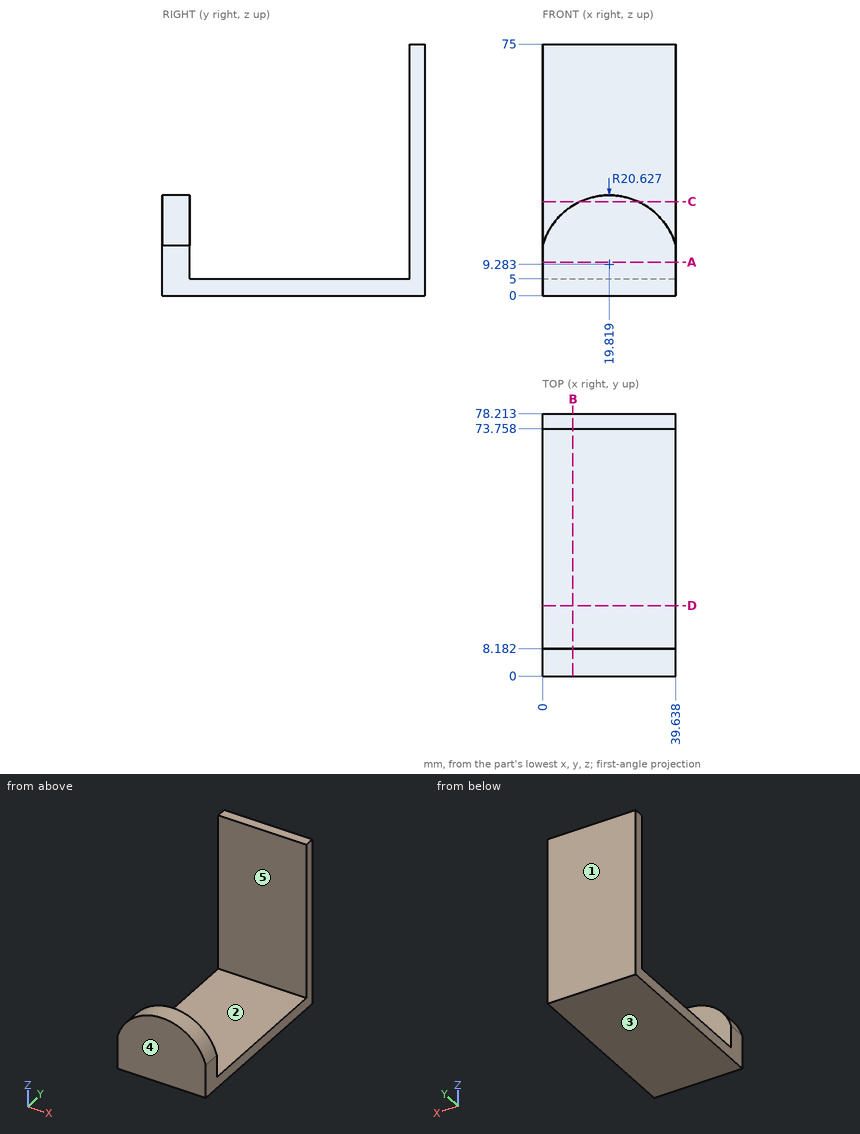
Geometry check sheet. Reference: drawing and pictorial views, mm from the part's lowest x, y, z. A direction names the side the tool comes from. Coordinates: 2 decimals unless noted, no trailing zeros. Order: outer loops, then holes, each group sorted by start corner. A loop starts at its lowest first (then second) coordinate and runs counter-clockwise, first axis right, second up. Notation, with made-up numbers: M -4.75,26.25 L 2.25,26.25 A28 ccw 2.25,63.25 Z; hole C -6,3 d9. An arc over 180 degrees is marked long. Return JSON: item names as keys, results as strings.
1) Cross-section at B-B, the plane x = 9. Record the boundary of the cut face in (y, z) (1 decimal).
Answer list:
{"outline": "M 0,0 L 78.2,0 L 78.2,75 L 73.8,75 L 73.8,5 L 8.2,5 L 8.2,26.8 L 0,26.8 Z"}
2) Cross-section at D-D, the plane y = 21. Record the boundary of the cut face in (x, z), and give its area (3 significant figures).
Answer list:
{"outline": "M 0,0 L 39.64,0 L 39.64,5 L 0,5 Z", "area": "198 mm2"}
3) Access from +Z, -Z, +X, -X, +Y, -Y to the whole of each face (thin tool, end or side, straight path). Record for the marked faces 1 and 2.
Answer list:
{"face 1": "+Z, -Z, +X, -X, +Y", "face 2": "+Z, +X, -X"}
4) Thickness scan on L1, parallel to Y at x = 19.5, z = 26.5; L2, parallel to Z at x = 21, y = 12; L3, parallel to Y at x = 26.5, z = 47.5. Record the ranges inside material, lowest first. Write a range as [from, to].
Answer list:
{"L1": "[0, 8.18], [73.76, 78.21]", "L2": "[0, 5]", "L3": "[73.76, 78.21]"}
5) Release check for a two-part mould opening along Y. For the marked faces 3, 4 and 5 record: +Y half, -Y half, draft (parallel to the pull), parting line (faces both ways), or undercut.
Answer list:
{"face 3": "draft", "face 4": "-Y half", "face 5": "undercut"}
6) Gauge pin test, flat end, axial feed: pin 1 (3 mm diameter, centred on x = 32.5, y = 26, fed in from +Z). Record the tip position at first contact, or that the pin passes through.
Answer list:
{"pin 1": "z = 5"}
7) Cross-section at C-C, the plane z = 28. Record the boundary of the cut face in (x, y).
Answer list:
{"outline": "M 0,73.76 L 39.64,73.76 L 39.64,78.21 L 0,78.21 Z; M 11.15,0 L 28.49,0 L 28.49,8.18 L 11.15,8.18 Z"}
8) Cross-section at A-A, the plane z = 10. Record the boundary of the cut face in (x, y), and give its area (3 significant figures).
Answer list:
{"outline": "M 0,0 L 39.64,0 L 39.64,8.18 L 0,8.18 Z; M 0,73.76 L 39.64,73.76 L 39.64,78.21 L 0,78.21 Z", "area": "501 mm2"}
